from build123d import *

# Parameters (mm, degrees)
CUT_EXTRUDE_1_DEPTH = 2
FILLET_1_R          = 0.3
CHAMFER_1_SIZE      = 1


with BuildPart() as part:
    # Эскиз1 → Повернуть1 (revolve)
    with BuildSketch(Plane.XY):
        with BuildLine():
            Line((0, 0), (0, 4))
            ThreePointArc((0, 4), (1.41886117, 4.74341649), (3, 5))
            Line((3, 5), (3.5, 5))
            Line((3.5, 5), (3.5, 3))
            Line((3.5, 3), (33.5, 3))
            Line((33.5, 3), (33.5, 0))
            Line((33.5, 0), (0, 0))
        make_face()
    revolve(axis=Axis((33.5, 0, 0), (-1, 0, 0)))

    # Эскиз2 → Вырез-Вытянуть1 (cut)
    with BuildSketch(Plane.ZY):
        Polygon((1.154700538, 2), (-1.154700538, 2), (-2.309401077, 0), (-1.154700538, -2), (1.154700538, -2), (2.309401077, 0), align=None)
    extrude(amount=-CUT_EXTRUDE_1_DEPTH, mode=Mode.SUBTRACT)

    # Скругление1
    fillet_1_edges = [part.edges().sort_by_distance(p)[0] for p in [
        (3.5, -3, 0),
        (3.5, -5, 0),
    ]]
    fillet(fillet_1_edges, radius=FILLET_1_R)

    # Фаска1
    chamfer_1_edges = [part.edges().sort_by_distance(p)[0] for p in [
        (33.5, -3, 0),
    ]]
    chamfer(chamfer_1_edges, length=CHAMFER_1_SIZE)


solid = part.part
Part model, mm, in its own coordinate system. A direction names the side the tool comes from. Coordinates: 2 decimals unless noted, no trailing zeros. Order: outer loops, then holes, each group sorted by start corner. A loop starts at its lowest first (then second) coordinate and runs counter-clockwise, first axis right, second up. Notation, with made-up numbers: M 40.5,75.5 L 56.5,75.5 A28 cw 56.5,106.5 Z; hole C 28.5,83 d7. An arc over 180 degrees is marked long. One line per question, with ' | ' between items.
Q1. Two-plate mould, pull along Z, no slides. Class faces 1 (the face through (0.986, -1.014, 1.724)), 2 (the face through (3.5, 2, 3)), 3 (the face through (18, -3, 0)): +Z half, -Z half, draft (parallel to the pull), parting line (faces both ways), or undercut.
A:
face 1: undercut | face 2: draft | face 3: parting line
Q2. 3-axis set-ups, long thin cutter, end or side, ignore diameter. For faces 4 (the face through (33.5, 0, 0)), 5 (the face through (1, 2, 0)): which of +Z, -Z, +X, -X, +Y, -Y reach the whole face in a straight line?
A:
face 4: +Z, -Z, +X, +Y, -Y | face 5: -X
Q3. Pin check, flat tips, straight feed: P1, Ø3, axis at x = 10.5, z = 2, coming from the -Y side; P2, Ø2, axis at x = 28, y = -2.5, coming from the +Z side; P3, Ø5, axis at x = 19.5, y = -3, coming from the +Z side; P4, Ø4.5, axis at y = -1, z = 2, coming from the +X side. Stop position of each tip, or through.
A:
P1: stops at y = -2.96 | P2: stops at z = 2.6 | P3: stops at z = 2.96 | P4: stops at x = 33.5
Q4. Drill centre lines: line 1 (X direction, y = -1.25, z = -3.75); line 2 (X direction, y = -1.5, z = -1); line 3 (Z direction, x = 5.5, y = 2.25). Where is each one in solid material? Low to high.
A:
line 1: x = 0 to 3.5 | line 2: x = 2 to 33.5 | line 3: z = -1.98 to 1.98
Q5. Slice it at B-B (x = 26.5). Give the cut face in (y, z), and give its area (3 significant figures).
A:
outline: C 0,0 d6 | area: 28.3 mm^2
Q6. Slice it at A-A (z = 0). Give the cut face in (x, y).
A:
outline: M 0,-4 A5 ccw 3,-5 L 3.2,-5 A0.3 ccw 3.5,-4.7 L 3.5,-3.3 A0.3 cw 3.8,-3 L 32.5,-3 L 33.5,-2 L 33.5,2 L 32.5,3 L 3.8,3 A0.3 cw 3.5,3.3 L 3.5,4.7 A0.3 ccw 3.2,5 L 3,5 A5 ccw 0,4 L 0,2 L 2,2 L 2,-2 L 0,-2 Z
